```python
from build123d import *

# Parameters (mm, degrees)
F0_W      = 44
F0_H      = 29
F1_DEPTH  = 1.5
F2_W      = 39
F2_H      = 24
F3_DEPTH  = 15
F5_DEPTH  = 13
F8_W      = 24
F8_H      = 2.0449477285
F9_DEPTH  = 39
F11_DEPTH = 12.4
F12_W     = 12.0227243644
F12_H     = 12.4
F13_DEPTH = 11


# Not quite as in the source:
# - a feature names something its author has since deleted; it is built from what else it names


with BuildPart() as f1:
    # F0 (on Top) → F1 (new body)
    with BuildSketch(Plane.XY):
        with Locations((7.5298845768, 8.4944772368)):
            Rectangle(F0_W, F0_H)
    extrude(amount=F1_DEPTH)

    # F2 (on face) → F3 (join)
    with BuildSketch(Plane.XY.offset(1.5)):
        with Locations((7.5298845768, 8.4944772368)):
            Rectangle(F2_W, F2_H)
    extrude(amount=F3_DEPTH)

    # F4 (on face) → F5 (cut)
    with BuildSketch(Plane.XY.offset(16.5)):
        Polygon((22.4261898547, 20.4944772368), (-11.9701154232, 20.4944772368), (-11.9701154232, -3.5055227632), (0, 4.4034305029), (-7.16903992, -3.5055227632), (27.0298845768, -3.5055227632), (14.4714023918, 4.4034305029), (27.0298845768, 0), (27.0298845768, 20.4944772368), (14.4714023918, 13.7267839164), align=None)
    extrude(amount=-F5_DEPTH, mode=Mode.SUBTRACT)

    # F8 (on face) → F9 (join)
    with BuildSketch(Plane(origin=(-11.9701154232, 0, 0), x_dir=(0, -1, 0), z_dir=(-1, 0, 0))):
        with Locations((-8.4944772368, 17.5224738643)):
            Rectangle(F8_W, F8_H)
    extrude(amount=-F9_DEPTH)

    # F10 (on face) → F11 (join)
    with BuildSketch(Plane.XY.offset(18.5449477285)):
        Polygon((16.0282067955, 20.4944772368), (-2.7732178569, 20.4944772368), (-11.9701154232, 11.2487543374), (-11.9701154232, 4.2380536906), (-2.7732178569, -3.5055227632), (27.0298845768, -3.5055227632), (27.0298845768, 11.2487543374), align=None)
    extrude(amount=F11_DEPTH)

    # F12 (on face) → F13 (join)
    with BuildSketch(Plane(origin=(-2.8775827287, -3.4176499389, 0), x_dir=(0.7649595289, -0.6440783486, 0), z_dir=(-0.6440783486, -0.7649595289, 0))):
        with Locations((-5.8749302955, 24.7449477285)):
            Rectangle(F12_W, F12_H)
    extrude(amount=F13_DEPTH)


solid = f1.part
```
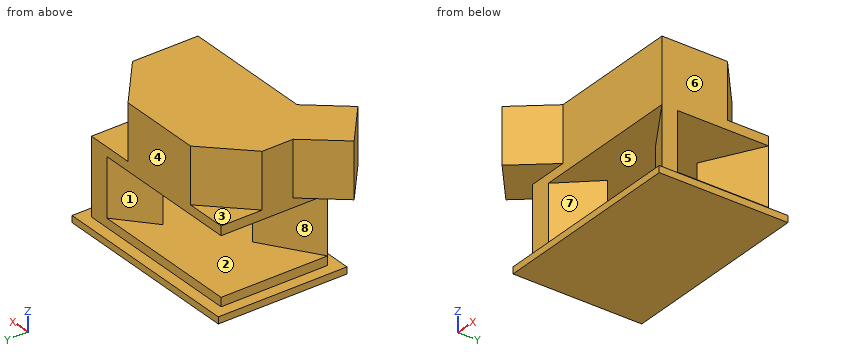
Design review of the part built by this model. Coordinates are the model's own, in mm. Face numbers are marked on the shaded views. A direction names the side the tool comes from. Give positions to 0.01 mm unless a question says otherwise; leave off trailing zeros. Write each loop counter-clockwise with the first axis right and the second up, starting at its lowest first coordinate (ties: lowest second). Pieces come first, ordered by that corner, then holes. Notation, with made-up numbers: (39, 67) -> (62, 67) arc R11 ccw to (62, 77) -> close; hole circle Ø10 at (6.5, 49.25). An arc over 180 degrees is marked (long way). Answer in a Markdown table with one row per item.
(1) Consider section D-D (z = 24.5). State the section outline as (x, y) points, then the cut area to 3 significant figures.
Results:
| item | result |
|---|---|
| outline | (-19.05, -4.18) -> (-9.86, -11.92) -> (-2.77, -3.51) -> (27.03, -3.51) -> (27.03, 11.25) -> (16.03, 20.49) -> (-2.77, 20.49) -> (-11.97, 11.25) -> (-11.97, 4.24) -> close |
| area | 939 mm2 |
(2) Consider section B-B (y = 7.5). State the section outline as (x, z) points.
Results:
| item | result |
|---|---|
| outline | (-14.47, 0) -> (29.53, 0) -> (29.53, 1.5) -> (27.03, 1.5) -> (27.03, 3.5) -> (-11.97, 3.5) -> (-11.97, 1.5) -> (-14.47, 1.5) -> close; (-11.97, 16.5) -> (27.03, 16.5) -> (27.03, 30.94) -> (-11.97, 30.94) -> close |
(3) To check wall thickness, follow probe 1 along Z at (x, y) = (18, 18); probe 2 along Z at (x, y) = (-13, -0.5); probe 3 along Y at (x, z) = (6, 3). State the ranges of each line that lie inside material, in increasing order.
Results:
| item | result |
|---|---|
| probe 1 | 0 to 3.5, 16.5 to 30.94 |
| probe 2 | 0 to 1.5, 18.54 to 30.94 |
| probe 3 | -3.51 to 20.49 |
(4) Consider section A-A (z = 4.5). State the section outline as (x, y) points, then the cut area to 3 significant figures.
Results:
| item | result |
|---|---|
| outline | (-11.97, -3.51) -> (-7.17, -3.51) -> (0, 4.4) -> close; (14.47, 4.4) -> (27.03, -3.51) -> (27.03, 0) -> close; (14.47, 13.73) -> (27.03, 20.49) -> (22.43, 20.49) -> close |
| area | 56.6 mm2 |
(5) Clearance check with flat-ended pins moving along their axes: pin 1 (1 mm diameter, centred on x = 17.5, y = -4.5, fed in from +Z); pin 2 (12 mm diameter, centred on y = 5.5, z = 17, fed in from +X); pin 3 (0.8 mm diameter, centred on x = 7, z = 1, fed in from -Y). State where each tip first meets the part, or that it passes through.
Results:
| item | result |
|---|---|
| pin 1 | z = 1.5 |
| pin 2 | x = 27.03 |
| pin 3 | y = -6.01 |
(6) For the marked faces 1, 2, 3 and 4, list the 3-axis set-ups (+Z, -Z, +X, -X, +Y, -Y) from which the entire face can be reached by the end or side of a thin tool; tool diameter is ignored.
Results:
| item | result |
|---|---|
| face 1 | -X, +Y |
| face 2 | none |
| face 3 | +Z, -X, +Y |
| face 4 | +Z, +X, -X, +Y |
(7) Consider section C-C (x = 10.5). State the section outline as (y, z) points, then the cut area to 3 significant figures.
Results:
| item | result |
|---|---|
| outline | (-6.01, 0) -> (22.99, 0) -> (22.99, 1.5) -> (20.49, 1.5) -> (20.49, 3.5) -> (-3.51, 3.5) -> (-3.51, 1.5) -> (-6.01, 1.5) -> close; (-3.51, 16.5) -> (20.49, 16.5) -> (20.49, 30.94) -> (-3.51, 30.94) -> close |
| area | 438 mm2 |
(8) Mouldability with a two-part tool opening along Y and no side actions: class the marked faces 5, 6, 7 and 8 as +Y half, -Y half, draft (parallel to the pull), parting line (faces both ways), or undercut.
Results:
| item | result |
|---|---|
| face 5 | undercut |
| face 6 | draft |
| face 7 | -Y half |
| face 8 | +Y half |
